from build123d import *

# Parameters (mm, degrees)
SKETCH1_W           = 32
SKETCH1_H           = 20
SKETCH1_W_2         = 29
SKETCH1_H_2         = 12
BOSS_EXTRUDE1_DEPTH = 10
SKETCH2_W           = 36
SKETCH2_H           = 24
SKETCH2_W_2         = 32
SKETCH2_H_2         = 20
BOSS_EXTRUDE2_DEPTH = 2
SKETCH3_W           = 5
SKETCH3_H           = 6
CUT_EXTRUDE2_DEPTH  = 24.832750576


with BuildPart() as part:
    # Sketch1 → Boss-Extrude1 (new body)
    with BuildSketch(Plane.XY):
        Rectangle(SKETCH1_W, SKETCH1_H)
        Rectangle(SKETCH1_W_2, SKETCH1_H_2, mode=Mode.SUBTRACT)
    extrude(amount=BOSS_EXTRUDE1_DEPTH)

    # Sketch2 → Boss-Extrude2 (add)
    with BuildSketch(Plane(origin=(0, 0, 0), x_dir=(-1, 0, 0), z_dir=(0, 0, -1))):
        Rectangle(SKETCH2_W, SKETCH2_H)
        Rectangle(SKETCH2_W_2, SKETCH2_H_2, mode=Mode.SUBTRACT)
    extrude(amount=-BOSS_EXTRUDE2_DEPTH)

    # Sketch3 → Cut-Extrude2 (cut, through all)
    with BuildSketch(Plane(origin=(0, 0, 0), x_dir=(-1, 0, 0), z_dir=(0, 0, -1))):
        with Locations((12, -9)):
            Rectangle(SKETCH3_W, SKETCH3_H)
    extrude(amount=-CUT_EXTRUDE2_DEPTH, mode=Mode.SUBTRACT)


solid = part.part
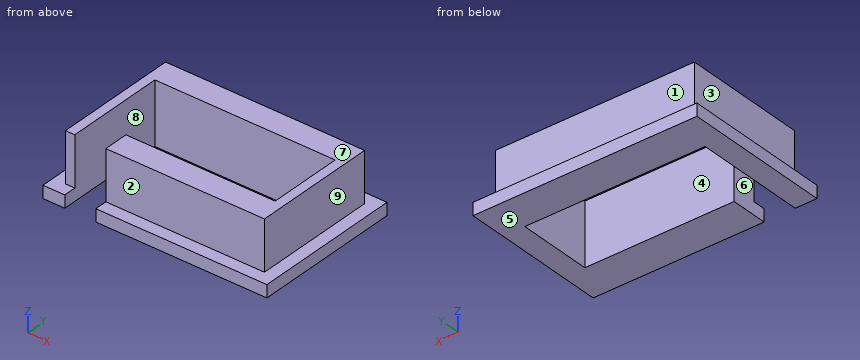
Model file for the job. Use its own axes, mm. Face numbers are marked on the shaded views. A direction names the side the tool comes from. Give positions to 0.01 mm unless a question says otherwise; leave off trailing zeros. Loops run counter-clockwise (first coordinate to the right, second up) from the corner with the lowest first, then second, coordinate; pieces in that order, holes last.
1) Pull direction X, two halves, no side cores. Call the marked faces 6, 7, 8 and 9: +X half, -X half, draft (parallel to the pull), parting line (faces both ways), or undercut.
2) Saw through at A-A (y = -0.75). Write the cut outline in (x, z).
3) Saw through at C-C (z = 1). Write the cut outline in (x, y), plus the area to 3 significant figures.
4) Wall check: line 1 (X direction, y = 2.75, z = 4.75); line 2 (Y direction, x = 11.5, z = 3.25); line 3 (X direction, y = -0.5, z = 1.5). Give the ranges that are in metal, low to high.
5) Saw through at B-B (x = 11.5). Write the cut outline in (y, z).
6) Saw through at D-D (y = 8.25). Write the cut outline in (x, z).
7) Tool access for the marked faces 1, 2, 3, 4 and 5: list every direction of +Z, -Z, +X, -X, +Y, -Y with a clear straight run to the whole face (end or side of a thin tool).
8) Flat gauge pins, fed straight in: pin 1 Ø0.8 at (x, z) = (-15, 5) entering from -Y; pin 2 Ø6 at (y, z) = (-1, 6.5) entering from -X; pin 3 Ø8 at (x, y) = (0.5, -5) entering from -Z. Where does each tip first touch, or does it go through?
Answer block:
1. face 6: undercut
1. face 7: draft
1. face 8: undercut
1. face 9: +X half
2. outline: (-18, 0) - (-14.5, 0) - (-14.5, 10) - (-16, 10) - (-16, 2) - (-18, 2) - close; (14.5, 0) - (18, 0) - (18, 2) - (16, 2) - (16, 10) - (14.5, 10) - close
3. outline: (-18, -12) - (-14.5, -12) - (-14.5, 6) - (14.5, 6) - (14.5, -6) - (-9.5, -6) - (-9.5, -12) - (18, -12) - (18, 12) - (-18, 12) - close
3. area: 486 mm2
4. line 1: x = -16 to -14.5, 14.5 to 16
4. line 2: y = -10 to -6, 6 to 10
4. line 3: x = -18 to -14.5, 14.5 to 18
5. outline: (-12, 0) - (-6, 0) - (-6, 10) - (-10, 10) - (-10, 2) - (-12, 2) - close; (6, 0) - (12, 0) - (12, 2) - (10, 2) - (10, 10) - (6, 10) - close
6. outline: (-18, 0) - (18, 0) - (18, 2) - (16, 2) - (16, 10) - (-16, 10) - (-16, 2) - (-18, 2) - close
7. face 1: +Z, +X, -X, +Y
7. face 2: +Z, +X, -X, -Y
7. face 3: +Z, -X, +Y, -Y
7. face 4: +Z, -Z
7. face 5: -Z, +X, -X, +Y, -Y
8. pin 1: stops at y = -10
8. pin 2: stops at x = -16
8. pin 3: stops at z = 0
